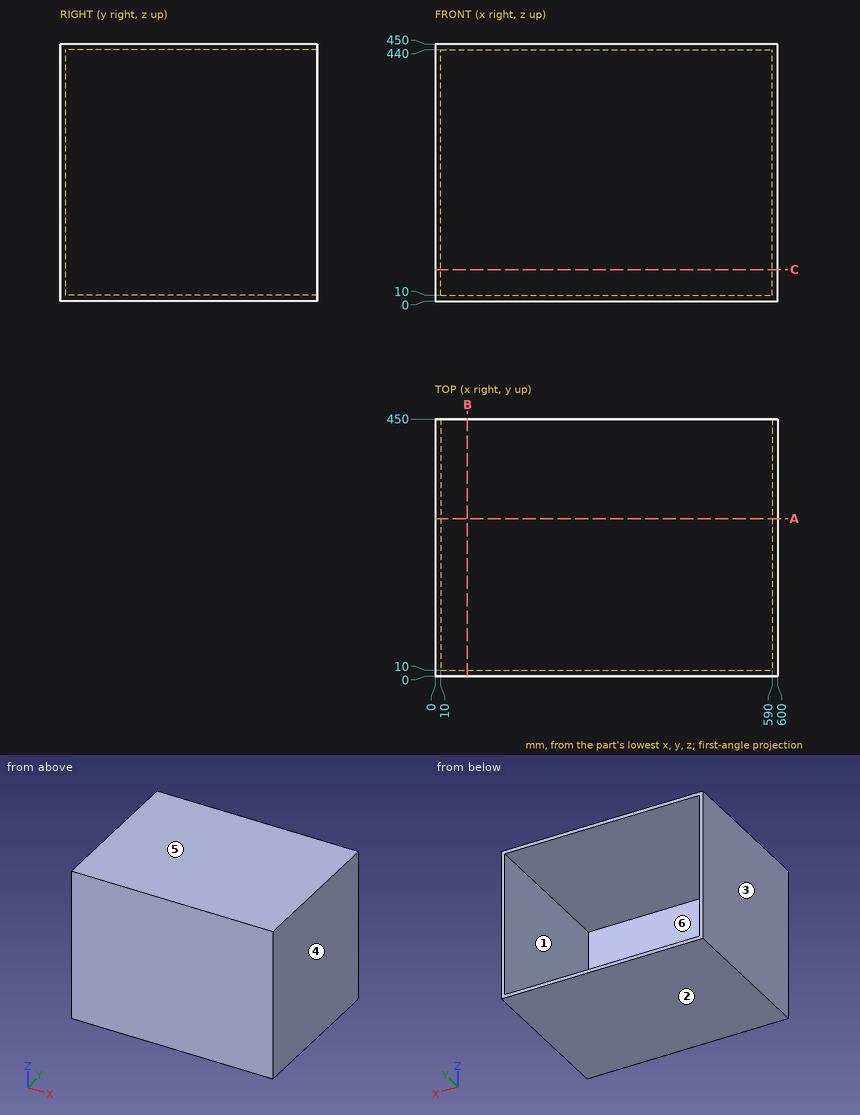
Answer from the drawing. Dimensions are ordinates in mm from the lowest x, y and z of the part. A direction names the side the tool comes from. Round coordinates to 2 decimals unless told otherwise and drop trailing zeros. Loops run counter-clockwise (first coordinate to the right, second up) from the corner with the lowest first, then second, coordinate; pieces in that order, holes last. Notation, with made-up numbers: (-9, 31) - (50, 31) arc R16 cw to (50, 48) - close; hole circle Ø5 at (36, -4). An arc over 180 degrees is marked (long way). Return JSON: item names as keys, results as strings. Group by question number.
1. Consider probe 1 along X at (y, z) = (319, 137.5); probe 2 along Z at (x, y) = (264, 403); probe 3 along Y at (x, z) = (522.5, 222). Determine where each line is inside the solid, lowest interval first.
2. Which of the six approach directions +Z, -Z, +X, -X, +Y, -Y give full straight-line access (tool end or side, diameter ignored) to the marked faces 5 and 6?
3. The part is cut by section A-A on y = 275.5. Determine the outline of the cut face in (x, z), then the cut area to 3 significant figures.
4. This flat-tipped pin is pushed along its axis until it touches: P1, Ø1.5, axis at x = 188.5, z = 269.5, coming from the +Y side. Where does it stop, or does it pass through?
5. The part is cut by section B-B on x = 56.5. Determine the outline of the cut face in (y, z), then the cut area to 3 significant figures.
6. The mould has two halves that part along X. Classify the marked faces 1, 2, 3 and 4: pulls with the +X half, pulls with the -X half, needs draft (parallel to the pull), parting line crosses it, or undercut.
7. The part is cut by section C-C on z = 55. Determine the outline of the cut face in (x, y), then the cut area to 3 significant figures.
Resolved:
{
 "1": {"probe 1": "x = 0 to 10, 590 to 600", "probe 2": "z = 0 to 10, 440 to 450", "probe 3": "y = 0 to 10"},
 "2": {"face 5": "+Z, +X, -X, +Y, -Y", "face 6": "+Y"},
 "3": {"outline": "(0, 0) - (600, 0) - (600, 450) - (0, 450) - close; hole (10, 10) - (590, 10) - (590, 440) - (10, 440) - close", "area": "20,600 mm²"},
 "4": {"P1": "stops at y = 10"},
 "5": {"outline": "(0, 0) - (450, 0) - (450, 10) - (10, 10) - (10, 440) - (450, 440) - (450, 450) - (0, 450) - close", "area": "13,300 mm²"},
 "6": {"face 1": "undercut", "face 2": "needs draft", "face 3": "pulls with the -X half", "face 4": "pulls with the +X half"},
 "7": {"outline": "(0, 0) - (600, 0) - (600, 450) - (590, 450) - (590, 10) - (10, 10) - (10, 450) - (0, 450) - close", "area": "14,800 mm²"}
}
